Work out the finished part from the listing and answer in its coordinate system (mm). Coordinates: 2 decimals unless noted, no trailing zeros. Loops run counter-clockwise (first coordinate to the right, second up) from the corner with the lowest first, then second, coordinate; pieces in that order, holes last. Notation, with made-up numbers: (60, -29) -> (92, -29) arc R11 ccw to (92, -16) -> close; hole circle Ø4 at (25.25, -7.75). An arc over 180 degrees is marked (long way). Use a Markdown table: item, result.
from build123d import *

# Parameters (mm, degrees)
SKETCH1_R           = 2.55
SKETCH1_R_2         = 3.6
BOSS_EXTRUDE1_DEPTH = 8.4


with BuildPart() as part:
    # Sketch1 → Boss-Extrude1 (new body)
    with BuildSketch(Plane(origin=(0, 0, 0), x_dir=(1, 0, 0), z_dir=(0, 1, 0))):
        with BuildLine():
            Line((29.75, -32.75), (-29.75, -32.75))
            ThreePointArc((-29.75, -32.75), (-31.871320344, -31.871320344), (-32.75, -29.75))
            Line((-32.75, -29.75), (-32.75, 29.75))
            ThreePointArc((-32.75, 29.75), (-31.871320344, 31.871320344), (-29.75, 32.75))
            Line((-29.75, 32.75), (29.75, 32.75))
            ThreePointArc((29.75, 32.75), (31.871320344, 31.871320344), (32.75, 29.75))
            Line((32.75, 29.75), (32.75, -29.75))
            ThreePointArc((32.75, -29.75), (31.871320344, -31.871320344), (29.75, -32.75))
        make_face()
        with Locations((0, 10)):
            Circle(SKETCH1_R, mode=Mode.SUBTRACT)
        Circle(SKETCH1_R, mode=Mode.SUBTRACT)
        with Locations((10, 0)):
            Circle(SKETCH1_R, mode=Mode.SUBTRACT)
        with Locations((-10, 0)):
            Circle(SKETCH1_R, mode=Mode.SUBTRACT)
        with Locations((-19.85, 20)):
            Circle(SKETCH1_R_2, mode=Mode.SUBTRACT)
        with Locations((-19.85, 0)):
            Circle(SKETCH1_R_2, mode=Mode.SUBTRACT)
        with Locations((-19.85, -20)):
            Circle(SKETCH1_R_2, mode=Mode.SUBTRACT)
        with Locations((-19.85, 10)):
            Circle(SKETCH1_R, mode=Mode.SUBTRACT)
        with Locations((19.85, 20)):
            Circle(SKETCH1_R, mode=Mode.SUBTRACT)
        with Locations((19.85, 0)):
            Circle(SKETCH1_R, mode=Mode.SUBTRACT)
        with Locations((19.85, -20)):
            Circle(SKETCH1_R, mode=Mode.SUBTRACT)
        with Locations((0, -10)):
            Circle(SKETCH1_R, mode=Mode.SUBTRACT)
        with Locations((19.85, 10)):
            Circle(SKETCH1_R, mode=Mode.SUBTRACT)
        with Locations((19.85, -10)):
            Circle(SKETCH1_R, mode=Mode.SUBTRACT)
        with Locations((-19.85, -10)):
            Circle(SKETCH1_R, mode=Mode.SUBTRACT)
        with BuildLine():
            Line((10.32, 17.5), (-10.32, 17.5))
            ThreePointArc((-10.32, 17.5), (-12.82, 20), (-10.32, 22.5))
            Line((-10.32, 22.5), (10.32, 22.5))
            ThreePointArc((10.32, 22.5), (12.82, 20), (10.32, 17.5))
        make_face(mode=Mode.SUBTRACT)
        with BuildLine():
            Line((3.25, 26.2), (-3.25, 26.2))
            ThreePointArc((-3.25, 26.2), (-4.75, 27.7), (-3.25, 29.2))
            Line((-3.25, 29.2), (3.25, 29.2))
            ThreePointArc((3.25, 29.2), (4.75, 27.7), (3.25, 26.2))
        make_face(mode=Mode.SUBTRACT)
        with BuildLine():
            Line((-16.9, 26.2), (-23.4, 26.2))
            ThreePointArc((-23.4, 26.2), (-24.9, 27.7), (-23.4, 29.2))
            Line((-23.4, 29.2), (-16.9, 29.2))
            ThreePointArc((-16.9, 29.2), (-15.4, 27.7), (-16.9, 26.2))
        make_face(mode=Mode.SUBTRACT)
        with BuildLine():
            Line((16.9, 26.2), (23.4, 26.2))
            ThreePointArc((23.4, 26.2), (24.9, 27.7), (23.4, 29.2))
            Line((23.4, 29.2), (16.9, 29.2))
            ThreePointArc((16.9, 29.2), (15.4, 27.7), (16.9, 26.2))
        make_face(mode=Mode.SUBTRACT)
        with BuildLine():
            Line((10.32, -17.5), (-10.32, -17.5))
            ThreePointArc((-10.32, -17.5), (-12.82, -20), (-10.32, -22.5))
            Line((-10.32, -22.5), (10.32, -22.5))
            ThreePointArc((10.32, -22.5), (12.82, -20), (10.32, -17.5))
        make_face(mode=Mode.SUBTRACT)
        with BuildLine():
            Line((-16.9, -26.2), (-23.4, -26.2))
            ThreePointArc((-23.4, -26.2), (-24.9, -27.7), (-23.4, -29.2))
            Line((-23.4, -29.2), (-16.9, -29.2))
            ThreePointArc((-16.9, -29.2), (-15.4, -27.7), (-16.9, -26.2))
        make_face(mode=Mode.SUBTRACT)
        with BuildLine():
            Line((3.25, -26.2), (-3.25, -26.2))
            ThreePointArc((-3.25, -26.2), (-4.75, -27.7), (-3.25, -29.2))
            Line((-3.25, -29.2), (3.25, -29.2))
            ThreePointArc((3.25, -29.2), (4.75, -27.7), (3.25, -26.2))
        make_face(mode=Mode.SUBTRACT)
        with BuildLine():
            Line((16.9, -26.2), (23.4, -26.2))
            ThreePointArc((23.4, -26.2), (24.9, -27.7), (23.4, -29.2))
            Line((23.4, -29.2), (16.9, -29.2))
            ThreePointArc((16.9, -29.2), (15.4, -27.7), (16.9, -26.2))
        make_face(mode=Mode.SUBTRACT)
    extrude(amount=BOSS_EXTRUDE1_DEPTH)


solid = part.part
Q1. Section C-C on z = 0 is taken. Determine the outline of the cut face in (x, y), and give its area (3 significant figures).
Solved:
| item | result |
|---|---|
| outline | (-32.75, 0) -> (-23.45, 0) -> (-23.45, 8.4) -> (-32.75, 8.4) -> close; (-16.25, 0) -> (-12.55, 0) -> (-12.55, 8.4) -> (-16.25, 8.4) -> close; (-7.45, 0) -> (-2.55, 0) -> (-2.55, 8.4) -> (-7.45, 8.4) -> close; (2.55, 0) -> (7.45, 0) -> (7.45, 8.4) -> (2.55, 8.4) -> close; (12.55, 0) -> (17.3, 0) -> (17.3, 8.4) -> (12.55, 8.4) -> close; (22.4, 0) -> (32.75, 0) -> (32.75, 8.4) -> (22.4, 8.4) -> close |
| area | 318 mm² |
Q2. Consider line 1 (X direction, y = 4.5, z = 20); line 2 (Z direction, x = -10, y = 6.5); line 3 (X direction, y = 5.5, z = 0). Determine where each line is inside the solid, lowest interval first. Write a range as [from, to].
Solved:
| item | result |
|---|---|
| line 1 | [-32.75, -23.45], [-16.25, -12.82], [12.82, 17.3], [22.4, 32.75] |
| line 2 | [-32.75, -22.5], [-17.5, -2.55], [2.55, 17.5], [22.5, 32.75] |
| line 3 | [-32.75, -23.45], [-16.25, -12.55], [-7.45, -2.55], [2.55, 7.45], [12.55, 17.3], [22.4, 32.75] |
Q3. Section A-A on x = 19.85 is taken. State how many separate pieces and enclosed holes the cut face has, and give its area (3 significant figures).
Solved:
| item | result |
|---|---|
| separate pieces | 8 |
| enclosed holes | 0 |
| area | 286 mm² |
Q4. Determine the mould class of faces 1 (the cylindrical face through (-12.024, 4.141, 1.552)), 2 (the flat face through (32.75, 4, 0)) for opening direction X: pulls with the +X half, pulls with the -X half, needs draft (parallel to the pull), parting line crosses it, or undercut.
Solved:
| item | result |
|---|---|
| face 1 | undercut |
| face 2 | pulls with the +X half |
Q5. Section B-B on z = 27.7 is taken. Determine the outline of the cut face in (x, y), and give its area (3 significant figures).
Solved:
| item | result |
|---|---|
| outline | (-32.75, 0) -> (-24.9, 0) -> (-24.9, 8.4) -> (-32.75, 8.4) -> close; (-15.4, 0) -> (-4.75, 0) -> (-4.75, 8.4) -> (-15.4, 8.4) -> close; (4.75, 0) -> (15.4, 0) -> (15.4, 8.4) -> (4.75, 8.4) -> close; (24.9, 0) -> (32.75, 0) -> (32.75, 8.4) -> (24.9, 8.4) -> close |
| area | 311 mm² |
Q6. Given pin 1 Ø6 at (x, z) = (18.5, -17.5) entering from -Y; pin 2 Ø3 at (x, z) = (19.85, -10) entering from +Y, each flat-ended and moving along its own axis, determine where each tip first touches the part or whether it passes through.
Solved:
| item | result |
|---|---|
| pin 1 | y = 0 |
| pin 2 | through |
